Input: part model. Units: mm. Frame: model coordinates. A direction names the side the tool comes from. Give positions to 0.01 mm unless a question says otherwise; leave off trailing zeros. Write each loop counter-clockwise with the first axis right and the second up, starting at its lowest first coordinate (ties: lowest second). Pieces come first, ordered by that corner, then holes. Notation, with made-up numbers: (66.5, -25.5) - (116.5, -25.5) arc R32 ccw to (116.5, 8.5) - close; hole circle Ø1 at (8.5, 53). An arc over 180 degrees is marked (long way). Answer as a JSON object with one key per item and string values. Group by question number.
from build123d import *

# Parameters (mm, degrees)
SKETCH1_R           = 22.2
BOSS_EXTRUDE1_DEPTH = 2
SKETCH2_R           = 11
BOSS_EXTRUDE2_DEPTH = 12
SKETCH2_2_R         = 11
BOSS_EXTRUDE3_DEPTH = 7
SKETCH3_R           = 4
BOSS_EXTRUDE4_DEPTH = 9
SKETCH4_R           = 2.75
CUT_EXTRUDE1_DEPTH  = 3.1


with BuildPart() as part:
    # Sketch1 → Boss-Extrude1 (new body)
    with BuildSketch(Plane(origin=(0, 0, 0), x_dir=(1, 0, 0), z_dir=(0, 1, 0))):
        Circle(SKETCH1_R)
    extrude(amount=BOSS_EXTRUDE1_DEPTH)

    # Sketch2 → Boss-Extrude2 (add)
    with BuildSketch(Plane(origin=(0, 2, 0), x_dir=(1, 0, 0), z_dir=(0, 1, 0))):
        Circle(SKETCH2_R)
    extrude(amount=BOSS_EXTRUDE2_DEPTH)

    # Sketch2_2 → Boss-Extrude3 (add)
    with BuildSketch(Plane(origin=(0, 2, 0), x_dir=(1, 0, 0), z_dir=(0, 1, 0))):
        Circle(SKETCH2_2_R)
    extrude(amount=-BOSS_EXTRUDE3_DEPTH)

    # Sketch3 → Boss-Extrude4 (add)
    with BuildSketch(Plane.XZ.offset(5)):
        Circle(SKETCH3_R)
    extrude(amount=BOSS_EXTRUDE4_DEPTH)

    # Sketch4 → Cut-Extrude1 (cut)
    with BuildSketch(Plane(origin=(0, 2, 0), x_dir=(1, 0, 0), z_dir=(0, 1, 0))):
        with Locations((0, -17.95)):
            Circle(SKETCH4_R)
        with Locations((-15.545155998, 8.975)):
            Circle(SKETCH4_R)
        with Locations((15.545155998, 8.975)):
            Circle(SKETCH4_R)
    extrude(amount=-CUT_EXTRUDE1_DEPTH, mode=Mode.SUBTRACT)


solid = part.part
1) Pin query (flat end, axial travel): P1, Ø2, axis at y = 3.5, z = 8.5, coming from the +X side; P2, Ø9, axis at x = 0, z = 17.95, coming from the -Y side; P3, Ø6, axis at y = 5.5, z = -10, coming from the -X side. Return the tip coordinate at first contact, or that it passes through.
2) Cut plane B-B on z = 0. Return the cut outline in (x, y), and give its area (3 significant figures).
3) Cut plane A-A on x = 0. Return the cut outline in (y, z).
4) Line query: line 1 along Z through (x, y) = (0, 0.45); line 2 along Y through (x, z) = (3, -11); line 3 along Y through (x, z) = (5, 3.5). Output: solid intervals per line, ascending. Write a range as from..to.
5) Cut plane C-C on z = 17.95. Return the cut outline in (x, y).
6) Reachability of faces 1 (the face through (11.93, 0.99, -18.72)), 2 (the face through (-2.38, 7.92, 10.74)), 3 (the face through (0, -5, 5)) from +Z, -Z, +X, -X, +Y, -Y: full face, straight path, thin tool, end or side. Return the list, or none.
7) Cut plane D-D on y = 4.5. Return the cut outline in (x, z), and give its area (3 significant figures).
8) Mould query, pull axis X, two halves, no side actions, for faces 4 (the face through (0, 14, 0)), 5 (the face through (-0.596, 1.014, 20.635)), 6 (the face through (-2.38, -2.46, 10.74)). Classes: +X half, -X half, draft (parallel to the pull), parting line (faces both ways), or undercut.
Filled in:
{
 "1": {"P1": "stops at x = 8.05", "P2": "stops at y = 0", "P3": "stops at x = -8.49"},
 "2": {"outline": "(-22.2, 0) - (-11, 0) - (-11, -5) - (-4, -5) - (-4, -14) - (4, -14) - (4, -5) - (11, -5) - (11, 0) - (22.2, 0) - (22.2, 2) - (11, 2) - (11, 14) - (-11, 14) - (-11, 2) - (-22.2, 2) - close", "area": "535 mm²"},
 "3": {"outline": "(-14, -4) - (-5, -4) - (-5, -11) - (0, -11) - (0, -22.2) - (2, -22.2) - (2, -11) - (14, -11) - (14, 11) - (2, 11) - (2, 15.2) - (0, 15.2) - (0, 11) - (-5, 11) - (-5, 4) - (-14, 4) - close; (0, 20.7) - (2, 20.7) - (2, 22.2) - (0, 22.2) - close"},
 "4": {"line 1": "z = -22.2..15.2, 20.7..22.2", "line 2": "y = 0..2", "line 3": "y = -5..14"},
 "5": {"outline": "(-13.06, 0) - (-2.75, 0) - (-2.75, 2) - (-13.06, 2) - close; (2.75, 0) - (13.06, 0) - (13.06, 2) - (2.75, 2) - close"},
 "6": {"face 1": "+Y, -Y", "face 2": "+Y", "face 3": "-Y"},
 "7": {"outline": "circle Ø22 at (0, 0)", "area": "380 mm²"},
 "8": {"face 4": "draft", "face 5": "undercut", "face 6": "parting line"}
}
